from build123d import *

# Parameters (mm, degrees)
ESQUISSE1_R        = 2
ESQUISSE1_W        = 5
ESQUISSE1_H        = 5
BOSS_EXTRU_1_DEPTH = 5


with BuildPart() as part:
    # Esquisse1 → Boss.-Extru.1 (new body)
    with BuildSketch(Plane.XY):
        Polygon((-105, 22.5), (-50, 22.5), (-50, 27.5), (-45, 27.5), (-45, 22.5), (-42, 22.5), (-42, 19.5), (-43.5, 19.5), (-43.5, 16.5), (-42, 16.5), (-42, 12.5), (-38, 12.5), (-38, 16.5), (-36.5, 16.5), (-36.5, 19.5), (-38, 19.5), (-38, 22.5), (-35, 22.5), (-35, 27.5), (-30, 27.5), (-30, 22.5), (35, 22.5), (35, 27.5), (40, 27.5), (40, 22.5), (43, 22.5), (43, 19.5), (41.5, 19.5), (41.5, 16.5), (43, 16.5), (43, 12.5), (47, 12.5), (47, 16.5), (48.5, 16.5), (48.5, 19.5), (47, 19.5), (47, 22.5), (50, 22.5), (50, 27.5), (55, 27.5), (55, 22.5), (85, 22.5), (85, -2.5), (90, -2.5), (90, -7.5), (85, -7.5), (85, -10.5), (82, -10.5), (82, -9), (79, -9), (79, -10.5), (75, -10.5), (75, -14.5), (79, -14.5), (79, -16), (82, -16), (82, -14.5), (85, -14.5), (85, -17.5), (90, -17.5), (90, -22.5), (85, -22.5), (85, -48.5), (55, -48.5), (55, -53.5), (50, -53.5), (50, -48.5), (47, -48.5), (47, -45.5), (48.5, -45.5), (48.5, -42.5), (47, -42.5), (47, -38.5), (43, -38.5), (43, -42.5), (41.5, -42.5), (41.5, -45.5), (43, -45.5), (43, -48.5), (40, -48.5), (40, -53.5), (35, -53.5), (35, -48.5), (-105, -48.5), (-105, -22.5), (-110, -22.5), (-110, -17.5), (-105, -17.5), (-105, -14.5), (-102, -14.5), (-102, -16), (-99, -16), (-99, -14.5), (-95, -14.5), (-95, -10.5), (-99, -10.5), (-99, -9), (-102, -9), (-102, -10.5), (-105, -10.5), (-105, -7.5), (-110, -7.5), (-110, -2.5), (-105, -2.5), align=None)
        Circle(ESQUISSE1_R, mode=Mode.SUBTRACT)
        with Locations((70, 0)):
            Circle(ESQUISSE1_R, mode=Mode.SUBTRACT)
        with Locations((0, -20)):
            Circle(ESQUISSE1_R, mode=Mode.SUBTRACT)
        with Locations((70, -20)):
            Circle(ESQUISSE1_R, mode=Mode.SUBTRACT)
        with Locations((0, -40)):
            Circle(ESQUISSE1_R, mode=Mode.SUBTRACT)
        with Locations((70, -40)):
            Circle(ESQUISSE1_R, mode=Mode.SUBTRACT)
        with Locations((-70, 0)):
            Circle(ESQUISSE1_R, mode=Mode.SUBTRACT)
        with Locations((-7.5, 0)):
            Rectangle(ESQUISSE1_W, ESQUISSE1_H, mode=Mode.SUBTRACT)
        with Locations((7.5, 0)):
            Rectangle(ESQUISSE1_W, ESQUISSE1_H, mode=Mode.SUBTRACT)
        with Locations((62.5, 0)):
            Rectangle(ESQUISSE1_W, ESQUISSE1_H, mode=Mode.SUBTRACT)
        with Locations((77.5, 0)):
            Rectangle(ESQUISSE1_W, ESQUISSE1_H, mode=Mode.SUBTRACT)
        with Locations((-7.5, -20)):
            Rectangle(ESQUISSE1_W, ESQUISSE1_H, mode=Mode.SUBTRACT)
        with Locations((7.5, -20)):
            Rectangle(ESQUISSE1_W, ESQUISSE1_H, mode=Mode.SUBTRACT)
        with Locations((62.5, -20)):
            Rectangle(ESQUISSE1_W, ESQUISSE1_H, mode=Mode.SUBTRACT)
        with Locations((77.5, -20)):
            Rectangle(ESQUISSE1_W, ESQUISSE1_H, mode=Mode.SUBTRACT)
        with Locations((-7.5, -40)):
            Rectangle(ESQUISSE1_W, ESQUISSE1_H, mode=Mode.SUBTRACT)
        with Locations((7.5, -40)):
            Rectangle(ESQUISSE1_W, ESQUISSE1_H, mode=Mode.SUBTRACT)
        with Locations((62.5, -40)):
            Rectangle(ESQUISSE1_W, ESQUISSE1_H, mode=Mode.SUBTRACT)
        with Locations((77.5, -40)):
            Rectangle(ESQUISSE1_W, ESQUISSE1_H, mode=Mode.SUBTRACT)
        with Locations((-77.5, 0)):
            Rectangle(ESQUISSE1_W, ESQUISSE1_H, mode=Mode.SUBTRACT)
        with Locations((-62.5, 0)):
            Rectangle(ESQUISSE1_W, ESQUISSE1_H, mode=Mode.SUBTRACT)
    extrude(amount=BOSS_EXTRU_1_DEPTH)


solid = part.part
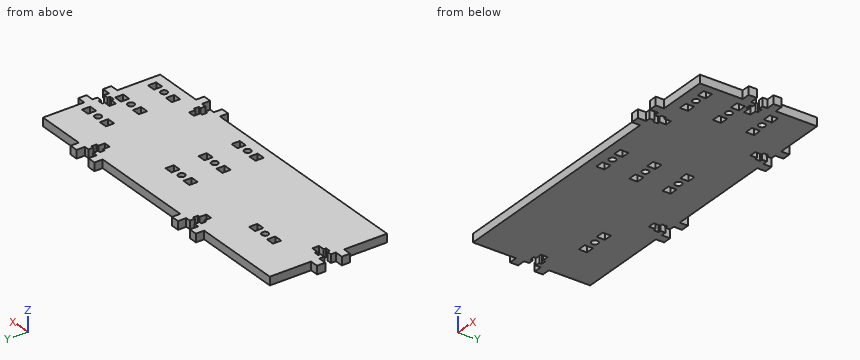
Can you work these out from the model? Positions are in its coordinate system, mm. Give positions to 0.01 mm unless a question says otherwise; leave off trailing zeros. Order: outer loops, then holes, each group sorted by start corner. A loop starts at its lowest first (then second) coordinate and runs counter-clockwise, first axis right, second up. Notation, with made-up numbers: M -4.5,-40 L 37.5,-40 A16 cw 37.5,-34 Z; hole C 16,59 d8. An arc over 180 degrees is marked long. Use one line per item in the form item = value. Start each with the question number.
Item 1: If we section it at D-D (y = 0): State how many separate pieces and enclosed holes the cut face has, then the cut area to 3 significant figures.
Item 2: If we section it at C-C (x = -70): Write out the boundary of the cut face in (y, z), then the cut area to 3 significant figures.
Item 3: If we section it at B-B (y = -20): Write out the boundary of the cut face in (x, z), then the cut area to 3 significant figures.
Item 4: If I drill on line 1 along Y through (x, z) = (70, 3.85); line 2 along X through (y, z) = (17.5, 1.8); line 3 along X through (y, z) = (-44, 1.8), over which ranges is the centre line in solid material (lowest first)?
Item 5: Will these pins go through, and if not, where does the flat tip stop? pin 1 Ø2.5 at (y, z) = (-0.5, 2.5) entering from +X; pin 2 Ø1.2 at (x, z) = (44.5, 2) entering from +Y; pin 3 Ø1.5 at (x, z) = (-106.5, 2) entering from -Y.
Item 6: If we section it at A-A (x = 0): Write out the boundary of the cut face in (y, z), then the cut area to 3 significant figures.
Outcome:
q1.separate_pieces = 10
q1.enclosed_holes = 0
q1.area = 740 mm2
q2.outline = M -48.5,0 L -2,0 L -2,5 L -48.5,5 Z; M 2,0 L 22.5,0 L 22.5,5 L 2,5 Z
q2.area = 335 mm2
q3.outline = M -110,0 L -10,0 L -10,5 L -110,5 Z; M -5,0 L -2,0 L -2,5 L -5,5 Z; M 2,0 L 5,0 L 5,5 L 2,5 Z; M 10,0 L 60,0 L 60,5 L 10,5 Z; M 65,0 L 68,0 L 68,5 L 65,5 Z; M 72,0 L 75,0 L 75,5 L 72,5 Z; M 80,0 L 90,0 L 90,5 L 80,5 Z
q3.area = 860 mm2
q4.line_1 = -48.5 to -42, -38 to -22, -18 to -2, 2 to 22.5
q4.line_2 = -105 to -43.5, -36.5 to 41.5, 48.5 to 85
q4.line_3 = -105 to 41.5, 48.5 to 85
q5.pin_1 = 85
q5.pin_2 = 12.5
q5.pin_3 = -22.5
q6.outline = M -48.5,0 L -42,0 L -42,5 L -48.5,5 Z; M -38,0 L -22,0 L -22,5 L -38,5 Z; M -18,0 L -2,0 L -2,5 L -18,5 Z; M 2,0 L 22.5,0 L 22.5,5 L 2,5 Z
q6.area = 295 mm2
